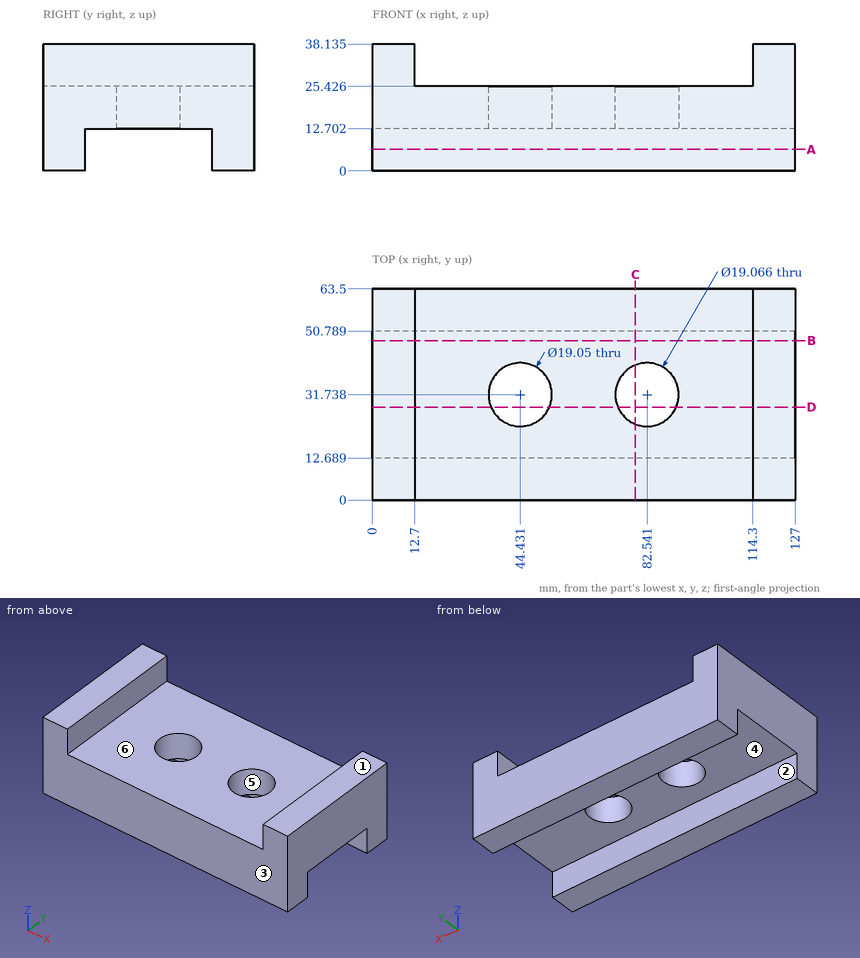
The drawing under review shows one solid part. Ordinate dimensions are in mm from its lowest x, y, z. A direction names the side the tool comes from. Coordinates: 2 decimals unless noted, no trailing zeros. Write each loop counter-clockwise with the first axis right and the second up, starting at its lowest first coordinate (ties: lowest second). Pieces come first, ordered by that corner, then holes. Notation, with made-up numbers: (-14, 25.25) - (13, 25.25) arc R20 cw to (13, 32.25) - close; hole circle Ø3 at (-39, -6.75). An arc over 180 degrees is marked (long way). Answer as CSV lines item,"result".
(1) Tool access review of the marked faces 4, 5 and 6: name each direction out of +Z, -Z, +X, -X, +Y, -Y from which nothing blocks a thin tool from reaching the whole face with its end or side.
Data:
face 4,"-Z, +X, -X"
face 5,"+Z, -Z"
face 6,"+Z, +Y, -Y"
(2) For line 1 along X through (y, z) = (35, 28.5); line 2 along Y through (x, z) = (47.5, 10.5); line 3 along Z through (x, y) = (17.5, 31.5), list the stretches that pass through material, from the lowest coordinate up. Write a range as [from, to].
Data:
line 1,"x = [0, 12.7], [114.3, 127]"
line 2,"y = [0, 12.69], [50.79, 63.5]"
line 3,"z = [12.7, 25.43]"
(3) We need section D-D (y = 28). Give the boundary of the cut face in (x, z) (1 decimal).
Data:
outline,"(0, 12.7) - (35.7, 12.7) - (35.7, 25.4) - (12.7, 25.4) - (12.7, 38.1) - (0, 38.1) - close; (53.2, 12.7) - (73.8, 12.7) - (73.8, 25.4) - (53.2, 25.4) - close; (91.3, 12.7) - (127, 12.7) - (127, 38.1) - (114.3, 38.1) - (114.3, 25.4) - (91.3, 25.4) - close"
(4) We need section B-B (y = 48). Give the boundary of the cut face in (x, z) (1 decimal), plus the area to 3 significant figures.
Data:
outline,"(0, 12.7) - (127, 12.7) - (127, 38.1) - (114.3, 38.1) - (114.3, 25.4) - (12.7, 25.4) - (12.7, 38.1) - (0, 38.1) - close"
area,"1,940 mm2"
(5) Mouldability with a two-part tool opening along Y and no side actions: class the marked faces 1, 2 and 3 as pulls with the +Y half, pulls with the -Y half, needs draft (parallel to the pull), parting line crosses it, or undercut.
Data:
face 1,"needs draft"
face 2,"undercut"
face 3,"pulls with the -Y half"
(6) Clearance check with flat-ended pins moving along their axes: pin 1 Ø12 at (x, y) = (39.5, 34) entering from -Z; pin 2 Ø4 at (y, z) = (21.5, 31) entering from -X; pin 3 Ø25 at (x, y) = (44.43, 31.74) entering from +Z. State where each tip first meets the part, or that it passes through.
Data:
pin 1,"stops at z = 12.7"
pin 2,"stops at x = 0"
pin 3,"stops at z = 25.43"
(7) We need section A-A (z = 6.5). Give the boundary of the cut face in (x, y).
Data:
outline,"(0, 0) - (127, 0) - (127, 12.69) - (0, 12.69) - close; (0, 50.79) - (127, 50.79) - (127, 63.5) - (0, 63.5) - close"
(8) We need section C-C (x = 79). Give the boundary of the cut face in (y, z).
Data:
outline,"(0, 0) - (12.69, 0) - (12.69, 12.7) - (22.89, 12.7) - (22.89, 25.43) - (0, 25.43) - close; (40.59, 12.7) - (50.79, 12.7) - (50.79, 0) - (63.5, 0) - (63.5, 25.43) - (40.59, 25.43) - close"
